Verification items for this drawing (mm, ordinates from the low corner). A direction names the side the tool comes from. Round coordinates to 2 decimals unless told otherwise and drop trailing zeros. Order: outer loops, then holes, each group sorted by start corner. A loop starts at its lowest first (then second) coordinate and runs counter-clockwise, first axis right, second up.
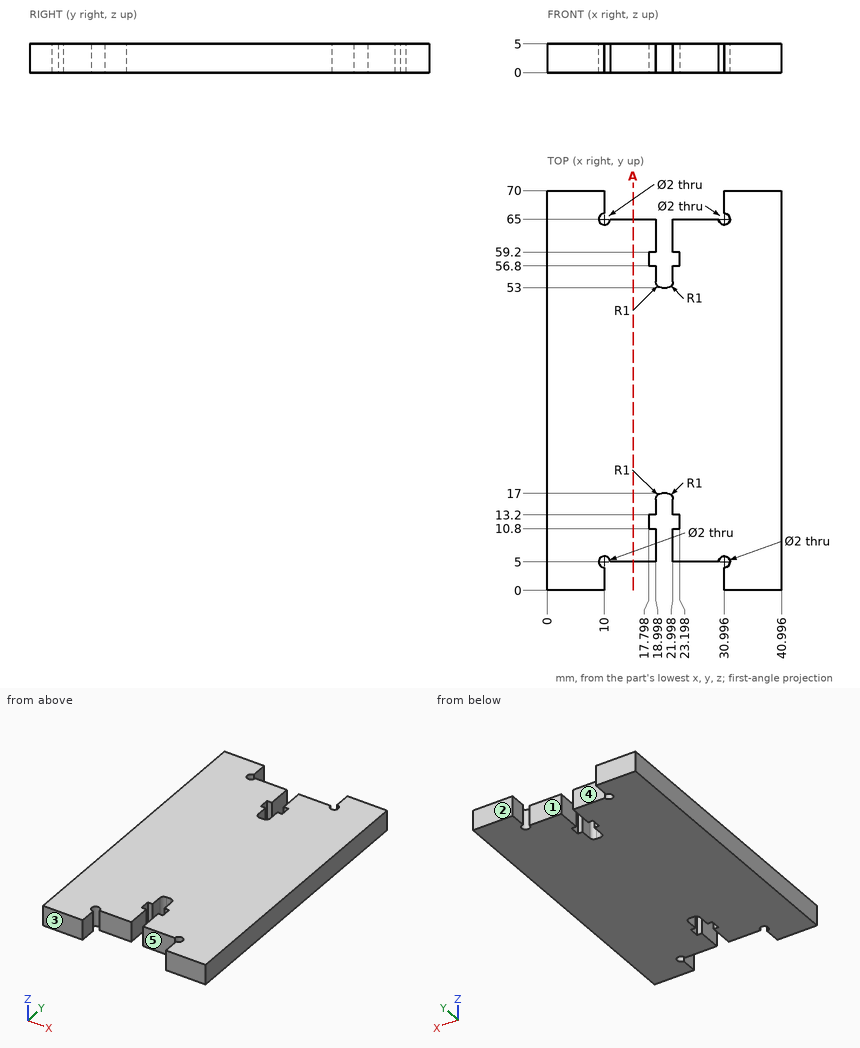
Item 1: Go/stop test with flat-tipped pins: P1, Ø0.6, axis at x = 18, z = 2, coming from the -Y side; P2, Ø1, axis at x = 11.5, z = 4.5, coming from the +Y side. Record where each tip stops, or that it passes through.
Answer:
P1: stops at y = 5
P2: stops at y = 65
Item 2: Scan lines: line 1 along Y through (x, z) = (9.5, 3.75); line 2 along X through (y, z) = (60.5, 2.6); line 3 along Y through (x, z) = (16, 2.85). Record each from-to range of solid material in increasing order.
Answer:
line 1: y = 0 to 4.13, 5.87 to 64.13, 65.87 to 70
line 2: x = 0 to 19, 22 to 41
line 3: y = 5 to 65
Item 3: Sectioned sample at A-A (x = 15). Record the cut outline in (y, z), and give its area (3 significant figures).
Answer:
outline: (5, 0) - (65, 0) - (65, 5) - (5, 5) - close
area: 300 mm2
Item 4: Release check for a two-part mould opening along X. For the marked faces 1 and 2 record: released by +X, released by -X, zero draft, split by the parting line, or undercut.
Answer:
face 1: undercut
face 2: zero draft
Item 5: Access from +Z, -Z, +X, -X, +Y, -Y to the whole of each face (thin tool, end or side, straight path). Record for the marked faces 3, 4 and 5.
Answer:
face 3: +Z, -Z, +X, -X, -Y
face 4: +Z, -Z, +Y
face 5: +Z, -Z, -Y
